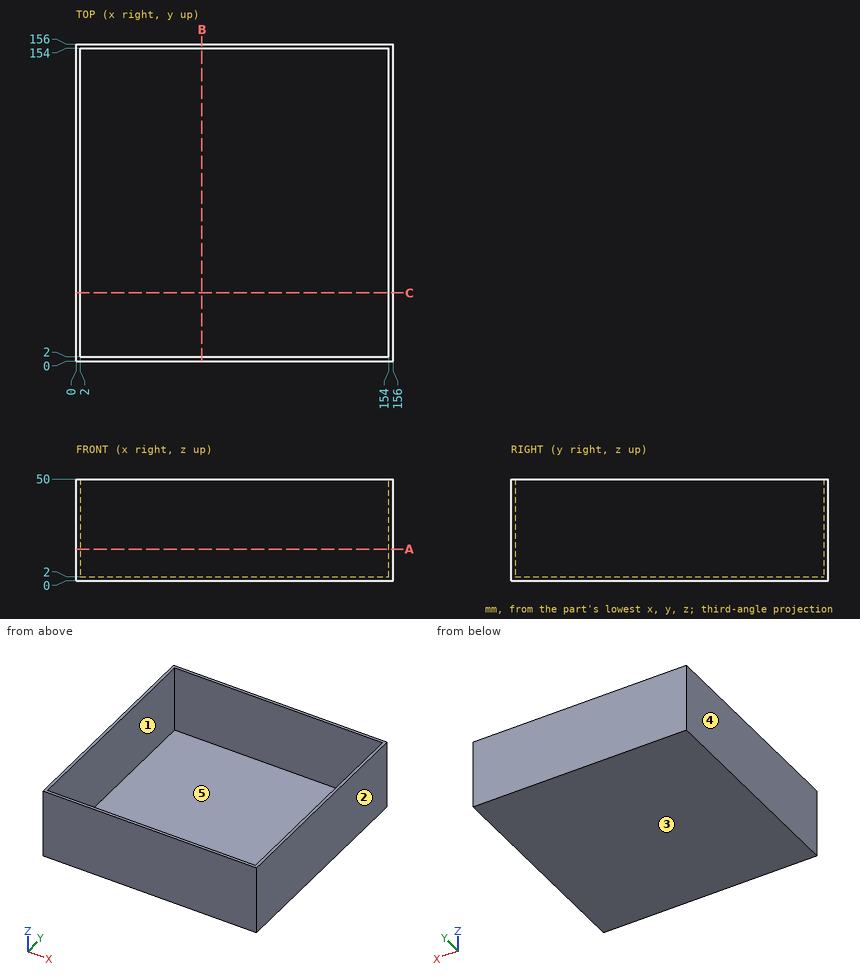
For this review, use the dimensioned drawing (mm, ordinates from the lowest corner) and the shaded views. A direction names the side the tool comes from. Coordinates: 2 decimals unless noted, no trailing zeros. Order: outer loops, then holes, each group sorted by start corner. A loop starts at its lowest first (then second) coordinate and runs counter-clockwise, first axis right, second up. Notation, with made-up numbers: (35, 24) -> (39, 24) arc R29 cw to (39, 60) -> close; hole circle Ø8 at (-16.5, -26.75). An arc over 180 degrees is marked (long way). One line per item, written item: value. Start each with the question number.
Q1. Mouldability with a two-part tool opening along X and no side actions: class the marked faces 1, 2 and 3 as pulls with the +X half, pulls with the -X half, needs draft (parallel to the pull), parting line crosses it, or undercut.
Q2. Insertion check: pin 1 Ø1 at (x, y) = (132.5, 51.5) entering from -Z. The pin has a flat end and moves straight along its axis. Give the tip position at first contact, or say it passes through.
Q3. Tool access review of the marked faces 4 and 5: name each direction out of +Z, -Z, +X, -X, +Y, -Y from which nothing blocks a thin tool from reaching the whole face with its end or side.
Q4. Take a section at A-A, the plane z = 15.5. State the section outline as (x, y) points, then the cut area to 3 significant figures.
Q5. For probe 1 along X at (y, z) = (104.5, 42.5); probe 2 along Z at (x, y) = (131.5, 90), list the stretches that pass through material, from the lowest coordinate up.
Q6. Take a section at B-B, the plane x = 62. State the section outline as (y, z) points, then the cut area to 3 significant figures.
Values follow:
1. face 1: undercut
1. face 2: pulls with the +X half
1. face 3: needs draft
2. pin 1: stops at z = 0
3. face 4: +Z, -Z, -X, +Y, -Y
3. face 5: +Z
4. outline: (0, 0) -> (156, 0) -> (156, 156) -> (0, 156) -> close; hole (2, 2) -> (154, 2) -> (154, 154) -> (2, 154) -> close
4. area: 1,230 mm2
5. probe 1: x = 0 to 2, 154 to 156
5. probe 2: z = 0 to 2
6. outline: (0, 0) -> (156, 0) -> (156, 50) -> (154, 50) -> (154, 2) -> (2, 2) -> (2, 50) -> (0, 50) -> close
6. area: 504 mm2
